```python
from build123d import *

# Parameters (mm, degrees)
SKIZZE1_W                                      = 300
SKIZZE1_H                                      = 300
SKIZZE1_R                                      = 3.25
AUFSATZ_LINEAR_AUSTRAGEN1_DEPTH                = 4
F_4_0_4_DURCHMESSER_BOHRUNG1_D                 = 4
M3_GEWINDEBOHRUNG1_AT_2_COUNT                  = 2
M3_GEWINDEBOHRUNG1_AT_2_PITCH                  = 7
SCHNITT_LINEAR_AUSTRAGEN2_REACH                = 426.283
SCHNITT_LINEAR_AUSTRAGEN4_REACH                = 426.283
KREISMUSTER1_COUNT                             = 3
SCHNITT_LINEAR_AUSTRAGEN3_REACH                = 426.283
FORMSENKUNG_F_R_M6_SENKSCHRAUBE_MIT_2_COUNT    = 2
FORMSENKUNG_F_R_M6_SENKSCHRAUBE_MIT_2_PITCH    = 280
F_4_3_4_3_DURCHMESSER_BOHRUNG1_D               = 4.3
FORMSENKUNG_F_R_M6_SENKSCHRAUBE_MIT_3_AT_COUNT = 2
FORMSENKUNG_F_R_M6_SENKSCHRAUBE_MIT_3_AT_PITCH = 280


with BuildPart() as part:
    # Skizze1 → Aufsatz-Linear austragen1 (new body)
    with BuildSketch(Plane.XY):
        with Locations((150, 150)):
            Rectangle(SKIZZE1_W, SKIZZE1_H)
        with Locations((150, 150)):
            Circle(SKIZZE1_R, mode=Mode.SUBTRACT)
    extrude(amount=AUFSATZ_LINEAR_AUSTRAGEN1_DEPTH)

    # Ø4.0 (4) Durchmesser Bohrung1 (through all)
    with Locations(Plane.XY.offset(4)):
        with Locations((160.25, 196.25), (170.25, 243.75), (160.25, 243.75), (170.25, 196.25)):
            f_4_0_4_durchmesser_bohrung1 = Hole(F_4_0_4_DURCHMESSER_BOHRUNG1_D / 2)

    # Skizze5 → M3 Gewindebohrung1 (revolve, cut)
    with BuildSketch(Plane(origin=(148.5, 262.5, 4), x_dir=(0, -1, 0), z_dir=(1, 0, 0))):
        Polygon((0, 0), (0, 9.251075774), (1.25, 8.5), (1.25, 0), align=None)
    m3_gewindebohrung1 = revolve(axis=Axis((148.5, 262.5, 10.35), (0, 0, -1)), mode=Mode.SUBTRACT)

    # M3 Gewindebohrung1 at 2: M3 Gewindebohrung1 ×2
    with Locations(*[(-i * M3_GEWINDEBOHRUNG1_AT_2_PITCH, 0, 0) for i in range(1, M3_GEWINDEBOHRUNG1_AT_2_COUNT)]):
        add(m3_gewindebohrung1, mode=Mode.SUBTRACT)

    # Skizze9 → Schnitt-Linear austragen2 (cut, up to next)
    with BuildSketch(Plane.XY.offset(4), mode=Mode.PRIVATE) as schnitt_linear_austragen2_sk1:
        with BuildLine():
            Line((139, 272.9), (151, 272.9))
            ThreePointArc((151, 272.9), (152.060660172, 272.460660172), (152.5, 271.4))
            Line((152.5, 271.4), (152.5, 266.9))
            ThreePointArc((152.5, 266.9), (152.060660172, 265.839339828), (151, 265.4))
            Line((151, 265.4), (139, 265.4))
            ThreePointArc((139, 265.4), (137.939339828, 265.839339828), (137.5, 266.9))
            Line((137.5, 266.9), (137.5, 271.4))
            ThreePointArc((137.5, 271.4), (137.939339828, 272.460660172), (139, 272.9))
        make_face()
    schnitt_linear_austragen2_tool1 = extrude(schnitt_linear_austragen2_sk1.sketch, amount=-SCHNITT_LINEAR_AUSTRAGEN2_REACH, mode=Mode.PRIVATE) & part.part
    schnitt_linear_austragen2 = schnitt_linear_austragen2_tool1.solids().sort_by_distance((145, 269.15, 4))[0]
    add(schnitt_linear_austragen2, mode=Mode.SUBTRACT)

    # Skizze16 → Schnitt-Linear austragen4 (cut, up to next)
    with BuildSketch(Plane.XY.offset(4), mode=Mode.PRIVATE) as schnitt_linear_austragen4_sk1:
        with BuildLine():
            Line((195, 227), (187, 227))
            ThreePointArc((187, 227), (186.292893219, 226.707106781), (186, 226))
            Line((186, 226), (186, 214))
            ThreePointArc((186, 214), (186.292893219, 213.292893219), (187, 213))
            Line((187, 213), (195, 213))
            ThreePointArc((195, 213), (195.707106781, 213.292893219), (196, 214))
            Line((196, 214), (196, 226))
            ThreePointArc((196, 226), (195.707106781, 226.707106781), (195, 227))
        make_face()
    schnitt_linear_austragen4_tool1 = extrude(schnitt_linear_austragen4_sk1.sketch, amount=-SCHNITT_LINEAR_AUSTRAGEN4_REACH, mode=Mode.PRIVATE) & part.part
    schnitt_linear_austragen4 = schnitt_linear_austragen4_tool1.solids().sort_by_distance((191, 220, 4))[0]
    add(schnitt_linear_austragen4, mode=Mode.SUBTRACT)

    # Kreismuster1: Ø4.0 (4) Durchmesser Bohrung1, M3 Gewindebohrung1, Schnitt-Linear austragen2, Schnitt-Linear austragen4 ×3 about axis
    kreismuster1_axis = Axis((150, 150, 0), (0, 0, 1))
    add([f_4_0_4_durchmesser_bohrung1.rotate(kreismuster1_axis, i * 360 / KREISMUSTER1_COUNT) for i in range(1, KREISMUSTER1_COUNT)], mode=Mode.SUBTRACT)
    add([m3_gewindebohrung1.rotate(kreismuster1_axis, i * 360 / KREISMUSTER1_COUNT) for i in range(1, KREISMUSTER1_COUNT)], mode=Mode.SUBTRACT)
    add([schnitt_linear_austragen2.rotate(kreismuster1_axis, i * 360 / KREISMUSTER1_COUNT) for i in range(1, KREISMUSTER1_COUNT)], mode=Mode.SUBTRACT)
    add([schnitt_linear_austragen4.rotate(kreismuster1_axis, i * 360 / KREISMUSTER1_COUNT) for i in range(1, KREISMUSTER1_COUNT)], mode=Mode.SUBTRACT)

    # Kreismuster1 copy 1 sketch → Kreismuster1 copy 1 (revolve, cut)
    with BuildSketch(Plane(origin=(56.822142074, 86.388784068, 4), x_dir=(0.8660254037844387, 0.4999999999999998, 0), z_dir=(-0.4999999999999998, 0.8660254037844387, 0))):
        Polygon((0, 0), (0, 9.251075774), (1.25, 8.5), (1.25, 0), align=None)
    revolve(axis=Axis((56.822142074, 86.388784068, 10.35), (0, 0, -1)), mode=Mode.SUBTRACT)

    # Kreismuster1 copy 2 sketch → Kreismuster1 copy 2 (revolve, cut)
    with BuildSketch(Plane(origin=(251.677857926, 101.111215932, 4), x_dir=(-0.8660254037844384, 0.5000000000000004, 0), z_dir=(-0.5000000000000004, -0.8660254037844384, 0))):
        Polygon((0, 0), (0, 9.251075774), (1.25, 8.5), (1.25, 0), align=None)
    revolve(axis=Axis((251.677857926, 101.111215932, 10.35), (0, 0, -1)), mode=Mode.SUBTRACT)

    # Skizze12 → Schnitt-Linear austragen3 (cut, up to next)
    with BuildSketch(Plane(origin=(0, 0, 0), x_dir=(-1, 0, 0), z_dir=(0, 0, -1)), mode=Mode.PRIVATE) as schnitt_linear_austragen3_sk1:
        with BuildLine():
            Line((-300, 17), (-300, 0))
            Line((-300, 0), (-283, 0))
            ThreePointArc((-283, 0), (-295.02081528, 4.97918472), (-300, 17))
        make_face()
    schnitt_linear_austragen3_tool1 = extrude(schnitt_linear_austragen3_sk1.sketch, amount=-SCHNITT_LINEAR_AUSTRAGEN3_REACH, mode=Mode.PRIVATE) & part.part
    # Skizze12 → Schnitt-Linear austragen3 (cut, up to next)
    with BuildSketch(Plane(origin=(0, 0, 0), x_dir=(-1, 0, 0), z_dir=(0, 0, -1)), mode=Mode.PRIVATE) as schnitt_linear_austragen3_sk2:
        with BuildLine():
            Line((-300, 300), (-280, 300))
            Line((-280, 300), (-280, 281))
            ThreePointArc((-280, 281), (-280.292893219, 280.292893219), (-281, 280))
            Line((-281, 280), (-300, 280))
            Line((-300, 280), (-300, 300))
        make_face()
    schnitt_linear_austragen3_tool2 = extrude(schnitt_linear_austragen3_sk2.sketch, amount=-SCHNITT_LINEAR_AUSTRAGEN3_REACH, mode=Mode.PRIVATE) & part.part
    # Skizze12 → Schnitt-Linear austragen3 (cut, up to next)
    with BuildSketch(Plane(origin=(0, 0, 0), x_dir=(-1, 0, 0), z_dir=(0, 0, -1)), mode=Mode.PRIVATE) as schnitt_linear_austragen3_sk3:
        with BuildLine():
            Line((0, 300), (-20, 300))
            Line((-20, 300), (-20, 281))
            ThreePointArc((-20, 281), (-19.707106781, 280.292893219), (-19, 280))
            Line((-19, 280), (0, 280))
            Line((0, 280), (0, 300))
        make_face()
    schnitt_linear_austragen3_tool3 = extrude(schnitt_linear_austragen3_sk3.sketch, amount=-SCHNITT_LINEAR_AUSTRAGEN3_REACH, mode=Mode.PRIVATE) & part.part
    # Skizze12 → Schnitt-Linear austragen3 (cut, up to next)
    with BuildSketch(Plane(origin=(0, 0, 0), x_dir=(-1, 0, 0), z_dir=(0, 0, -1)), mode=Mode.PRIVATE) as schnitt_linear_austragen3_sk4:
        with BuildLine():
            Line((-17, 0), (0, 0))
            Line((0, 0), (0, 17))
            ThreePointArc((0, 17), (-4.97918472, 4.97918472), (-17, 0))
        make_face()
    schnitt_linear_austragen3_tool4 = extrude(schnitt_linear_austragen3_sk4.sketch, amount=-SCHNITT_LINEAR_AUSTRAGEN3_REACH, mode=Mode.PRIVATE) & part.part
    add(schnitt_linear_austragen3_tool1.solids().sort_by_distance((296.202745, 3.797255, 0))[0], mode=Mode.SUBTRACT)
    add(schnitt_linear_austragen3_tool2.solids().sort_by_distance((290.005248, 290.005248, 0))[0], mode=Mode.SUBTRACT)
    add(schnitt_linear_austragen3_tool3.solids().sort_by_distance((9.994752, 290.005248, 0))[0], mode=Mode.SUBTRACT)
    add(schnitt_linear_austragen3_tool4.solids().sort_by_distance((3.797255, 3.797255, 0))[0], mode=Mode.SUBTRACT)

    # Skizze14 → Formsenkung f_r M6 Senkschraube mit Schl (revolve, cut)
    with BuildSketch(Plane(origin=(290, 10, 0), x_dir=(0, 1, 0), z_dir=(1, 0, 0))):
        Polygon((0, 0), (0, 4), (3.2, 4), (3.2, 3.1), (6.3, 0), align=None)
    formsenkung_f_r_m6_senkschraube_mit_schl = revolve(axis=Axis((290, 10, -6.35), (0, 0, 1)), mode=Mode.SUBTRACT)

    # Formsenkung f_r M6 Senkschraube mit  2: Formsenkung f_r M6 Senkschraube mit Schl ×2
    with Locations(*[(-i * FORMSENKUNG_F_R_M6_SENKSCHRAUBE_MIT_2_PITCH, 0, 0) for i in range(1, FORMSENKUNG_F_R_M6_SENKSCHRAUBE_MIT_2_COUNT)]):
        add(formsenkung_f_r_m6_senkschraube_mit_schl, mode=Mode.SUBTRACT)

    # Ø4.3 (4.3) Durchmesser Bohrung1 (through all)
    with Locations(Plane.XY.offset(4)):
        with Locations((30, 290), (110, 290), (190, 290), (270, 290)):
            Hole(F_4_3_4_3_DURCHMESSER_BOHRUNG1_D / 2)

    # Skizze19 → Formsenkung f_r M6 Senkschraube mit  3 (revolve, cut)
    with BuildSketch(Plane(origin=(10, 80, 4), x_dir=(0, -1, 0), z_dir=(1, 0, 0))):
        Polygon((0, 0), (0, 4), (3.2, 4), (3.2, 3.1), (6.3, 0), align=None)
    formsenkung_f_r_m6_senkschraube_mit_3 = revolve(axis=Axis((10, 80, 10.35), (0, 0, -1)), mode=Mode.SUBTRACT)

    # Formsenkung f_r M6 Senkschraube mit 3 at: Formsenkung f_r M6 Senkschraube mit  3 ×2
    with Locations(*[(i * FORMSENKUNG_F_R_M6_SENKSCHRAUBE_MIT_3_AT_PITCH, 0, 0) for i in range(1, FORMSENKUNG_F_R_M6_SENKSCHRAUBE_MIT_3_AT_COUNT)]):
        add(formsenkung_f_r_m6_senkschraube_mit_3, mode=Mode.SUBTRACT)


solid = part.part
```
Input: part model. Units: mm. Frame: model coordinates. Round coordinates to 2 decimals unless told otherwise and drop trailing zeros. One line per item, written item: value. Start each with the question number.
(1) Ray query, line 1 (X direction, y = 290, z = 1); line 2 (Y direction, x = 141.5, z = 1.8); line 3 (X direction, y = 218, z = 2.25). Return the intervals inside material, ascending. Write a range as [from, to].
(2) Contact query for a flat-ended pin moving along its axis: P1, Ø8.5, axis at x = 290, y = 10, coming from the -Z side. Output: stop coordinate, or through.
(3) Section A-A, the plane z = 2.1. Count the separate pieces of the cut face and the enclosed holes in it, plus the area to 3 significant figures.
(4) Draft query along Y for faces 1 (the cylindrical face through (12.839, 78.523, 0.456)), 2 (the cylindrical face through (294.89, 4.85, 1.97)), 3 (the conical face through (12.065, 7.307, 2.906)), 4 (the flat face through (148, 119, 4)). Return one class per face: +Y half, -Y half, draft (parallel to the pull), parting line (faces both ways), or undercut.
Results below:
1. line 1: [20, 27.85], [32.15, 107.85], [112.15, 187.85], [192.15, 267.85], [272.15, 280]
1. line 2: [0, 261.25], [263.75, 265.4], [272.9, 300]
1. line 3: [0, 186], [196, 300]
2. P1: z = 2.05
3. separate pieces: 1
3. enclosed holes: 33
3. area: 87,800 mm^2
4. face 1: undercut
4. face 2: -Y half
4. face 3: undercut
4. face 4: draft
